For this review, take the finished solid that the model builds, in its own axes (mm). Give positions to 0.01 mm unless a question says otherwise; leave off trailing zeros. Order: outer loops, then holes, each group sorted by start corner. A loop starts at its lowest first (then second) coordinate and runs counter-clockwise, first axis right, second up.
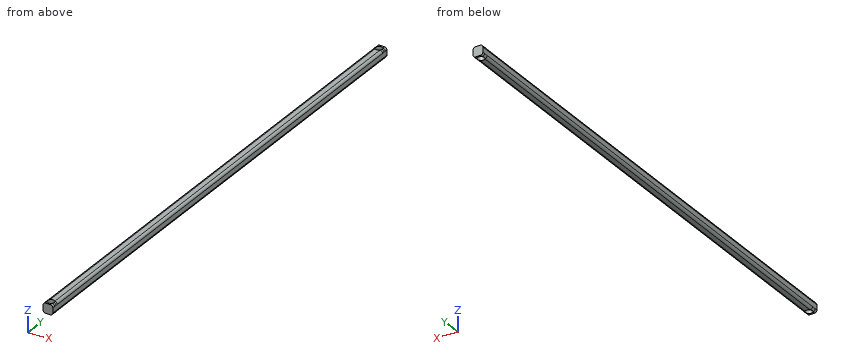
Autodesk Inventor part; units mm, degrees
ref_plane "YZ Plane" through (0, 0, 0) normal (1, 0, 0) x (0, 1, 0)
ref_plane "XZ Plane" through (0, 0, 0) normal (0, 1, 0) x (-1, 0, 0)
ref_plane "XY Plane" through (0, 0, 0) normal (0, 0, 1) x (1, 0, 0)
sketch "Sketch1" plane through (0, 0, 0) normal (0, 0, 1) x (1, 0, 0)
  line L0 (3.175, 171.45) -> (-3.175, 171.45)
  line L1 (-3.175, 171.45) -> (-3.175, -171.45)
  line L2 (-3.175, -171.45) -> (3.175, -171.45)
  line L3 (3.175, -171.45) -> (3.175, 171.45)
  line L4 (3.175, 171.45) -> (-3.175, -171.45) construction
  line L5 (-3.175, 171.45) -> (3.175, -171.45) construction
  circle A0 centre (0, -168.275) radius 2.1082
  circle A1 centre (0, 168.275) radius 2.1082
  point P0 (0, 0)
  dimension "d0" = 6.35
  dimension "d1" = 342.9
  dimension "d2" = 4.2164
  dimension "d3" = 3.175
  dimension "d4" = 4.2164
  dimension "d5" = 3.175
extrude "Extrusion1" add sketch "Sketch1" along normal blind 6.35
fillet "Fillet1" radius 1.5875 4 edges at (3.175, 0, 0) (3.175, 0, 6.35) (-3.175, 0, 0) (-3.175, 0, 6.35)
properties part number "Blocker B" material "Stainless Steel"
1) To check wall thickness, follow line 1 (Y direction, x = 0, z = 3.5); line 2 (Y direction, x = -1.75, z = 6); line 3 (X direction, y = -111, z = 5). State the ranges of each line that lie inside material, in increasing order.
Answer sheet:
line 1: y = -171.45 to -170.38, -166.17 to 166.17, 170.38 to 171.45
line 2: y = -171.45 to -169.45, -167.1 to 167.1, 169.45 to 171.45
line 3: x = -3.16 to 3.16
2) We need section A-A on x = 0. Give the boundary of the cut face in (y, z).
Answer sheet:
outline: (-171.45, 0) - (-170.38, 0) - (-170.38, 6.35) - (-171.45, 6.35) - close; (-166.17, 0) - (166.17, 0) - (166.17, 6.35) - (-166.17, 6.35) - close; (170.38, 0) - (171.45, 0) - (171.45, 6.35) - (170.38, 6.35) - close
3) Clearance check with a flat-ended pin moving along its axis: pin 1 (2.5 mm diameter, centred on x = 0, y = -168.275, fed in from -Z). State where the tip first meets the part, or that it passes through.
Answer sheet:
pin 1: passes through
